Build history of the part. All positions in model axes, mm. Face numbers are marked on the shaded views. Round coordinates to 2 decimals unless told otherwise and drop trailing zeros. Write each loop counter-clockwise with the first axis right and the second up, starting at its lowest first coordinate (ties: lowest second). Pieces come first, ordered by that corner, then holes. Notation, with made-up numbers: (72.25, -7.5) -> (131.25, -7.5) arc R23 cw to (131.25, 1.5) -> close; hole circle Ø9 at (-34.75, 30.25). An arc over 180 degrees is marked (long way). Answer in a Markdown table with one row per item.
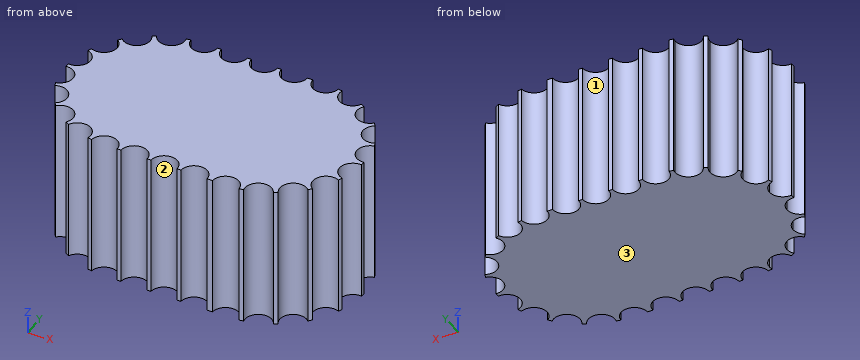
```python
from build123d import *

# Parameters (mm, degrees)
F1_DEPTH = 50.8


with BuildPart() as f1:
    # F0 (on Top) → F1 (new body)
    with BuildSketch(Plane.XY):
        with BuildLine():
            ThreePointArc((-39.4843, 31.75), (-44.0680803662, 26.9908545365), (-48.9958865795, 31.3928125))
            ThreePointArc((-48.9958865795, 31.3928125), (-49.7601296409, 31.2676461581), (-50.5210926164, 31.1238775246))
            ThreePointArc((-50.5210926164, 31.1238775246), (-50.3880618617, 30.485653166), (-50.3434395506, 29.83524071))
            ThreePointArc((-50.3434395506, 29.83524071), (-54.1035181326, 25.1794316985), (-59.4464558449, 27.8753109794))
            ThreePointArc((-59.4464558449, 27.8753109794), (-60.1218, 27.4963065702), (-60.7876995241, 27.1009435801))
            ThreePointArc((-60.7876995241, 27.1009435801), (-60.1220470195, 25.7816931615), (-59.8928066075, 24.321911069))
            ThreePointArc((-59.8928066075, 24.321911069), (-62.859641473, 19.9109029105), (-68.0637222924, 20.9956355589))
            ThreePointArc((-68.0637222924, 20.9956355589), (-68.568711069, 20.4085066075), (-69.0592298315, 19.8092358726))
            ThreePointArc((-69.0592298315, 19.8092358726), (-67.5322058816, 18.0997969887), (-66.9806065702, 15.875))
            ThreePointArc((-66.9806065702, 15.875), (-69.2087580954, 11.8428189452), (-73.808316411, 11.5835766274))
            ThreePointArc((-73.808316411, 11.5835766274), (-74.08204071, 10.8591395506), (-74.3380149087, 10.1282419657))
            ThreePointArc((-74.3380149087, 10.1282419657), (-71.7538504556, 8.4355421952), (-70.7519461581, 5.5133296409))
            ThreePointArc((-70.7519461581, 5.5133296409), (-72.3184192392, 1.9824914708), (-75.987355369, 0.7743673992))
            ThreePointArc((-75.987355369, 0.7743673992), (-75.9968, 0), (-75.987355369, -0.7743673992))
            ThreePointArc((-75.987355369, -0.7743673992), (-72.3184192392, -1.9824914708), (-70.7519461581, -5.5133296409))
            ThreePointArc((-70.7519461581, -5.5133296409), (-71.7538504556, -8.4355421952), (-74.3380149087, -10.1282419657))
            ThreePointArc((-74.3380149087, -10.1282419657), (-74.08204071, -10.8591395506), (-73.808316411, -11.5835766274))
            ThreePointArc((-73.808316411, -11.5835766274), (-69.2087580954, -11.8428189452), (-66.9806065702, -15.875))
            ThreePointArc((-66.9806065702, -15.875), (-67.5322058816, -18.0997969887), (-69.0592298315, -19.8092358726))
            ThreePointArc((-69.0592298315, -19.8092358726), (-68.568711069, -20.4085066075), (-68.0637222924, -20.9956355589))
            ThreePointArc((-68.0637222924, -20.9956355589), (-62.859641473, -19.9109029105), (-59.8928066075, -24.321911069))
            ThreePointArc((-59.8928066075, -24.321911069), (-60.1220470195, -25.7816931615), (-60.7876995241, -27.1009435801))
            ThreePointArc((-60.7876995241, -27.1009435801), (-60.1218, -27.4963065702), (-59.4464558449, -27.8753109794))
            ThreePointArc((-59.4464558449, -27.8753109794), (-54.1035181326, -25.1794316985), (-50.3434395506, -29.83524071))
            ThreePointArc((-50.3434395506, -29.83524071), (-50.3880618617, -30.485653166), (-50.5210926164, -31.1238775246))
            ThreePointArc((-50.5210926164, -31.1238775246), (-49.7601296409, -31.2676461581), (-48.9958865795, -31.3928125))
            ThreePointArc((-48.9958865795, -31.3928125), (-44.0680803662, -26.9908545365), (-39.4843, -31.75))
            Line((-39.4843, -31.75), (-38.0873, -31.75))
            ThreePointArc((-38.0873, -31.75), (-33.3248, -26.9875), (-28.5623, -31.75))
            Line((-28.5623, -31.75), (-27.1653, -31.75))
            ThreePointArc((-27.1653, -31.75), (-22.4028, -26.9875), (-17.6403, -31.75))
            Line((-17.6403, -31.75), (-16.2433, -31.75))
            ThreePointArc((-16.2433, -31.75), (-11.4808, -26.9875), (-6.7183, -31.75))
            Line((-6.7183, -31.75), (-4.7625, -31.75))
            ThreePointArc((-4.7625, -31.75), (-0.1787196338, -26.9908545365), (4.7490865795, -31.3928125))
            ThreePointArc((4.7490865795, -31.3928125), (5.5133296409, -31.2676461581), (6.2742926164, -31.1238775246))
            ThreePointArc((6.2742926164, -31.1238775246), (9.230268618, -25.3599546035), (15.1996558449, -27.8753109794))
            ThreePointArc((15.1996558449, -27.8753109794), (15.875, -27.4963065702), (16.5408995241, -27.1009435801))
            ThreePointArc((16.5408995241, -27.1009435801), (17.3472306164, -20.6736244087), (23.8169222924, -20.9956355589))
            ThreePointArc((23.8169222924, -20.9956355589), (24.321911069, -20.4085066075), (24.8124298315, -19.8092358726))
            ThreePointArc((24.8124298315, -19.8092358726), (23.3718605846, -13.49375), (29.561516411, -11.5835766274))
            ThreePointArc((29.561516411, -11.5835766274), (29.83524071, -10.8591395506), (30.0912149087, -10.1282419657))
            ThreePointArc((30.0912149087, -10.1282419657), (26.5774992344, -4.6863301948), (31.740555369, -0.7743673992))
            ThreePointArc((31.740555369, -0.7743673992), (31.75, 0), (31.740555369, 0.7743673992))
            ThreePointArc((31.740555369, 0.7743673992), (26.5774992344, 4.6863301948), (30.0912149087, 10.1282419657))
            ThreePointArc((30.0912149087, 10.1282419657), (29.83524071, 10.8591395506), (29.561516411, 11.5835766274))
            ThreePointArc((29.561516411, 11.5835766274), (23.3718605846, 13.49375), (24.8124298315, 19.8092358726))
            ThreePointArc((24.8124298315, 19.8092358726), (24.321911069, 20.4085066075), (23.8169222924, 20.9956355589))
            ThreePointArc((23.8169222924, 20.9956355589), (17.3472306164, 20.6736244087), (16.5408995241, 27.1009435801))
            ThreePointArc((16.5408995241, 27.1009435801), (15.875, 27.4963065702), (15.1996558449, 27.8753109794))
            ThreePointArc((15.1996558449, 27.8753109794), (9.230268618, 25.3599546035), (6.2742926164, 31.1238775246))
            ThreePointArc((6.2742926164, 31.1238775246), (5.5133296409, 31.2676461581), (4.7490865795, 31.3928125))
            ThreePointArc((4.7490865795, 31.3928125), (-0.1787196338, 26.9908545365), (-4.7625, 31.75))
            Line((-4.7625, 31.75), (-6.7183, 31.75))
            ThreePointArc((-6.7183, 31.75), (-11.4808, 26.9875), (-16.2433, 31.75))
            Line((-16.2433, 31.75), (-17.6403, 31.75))
            ThreePointArc((-17.6403, 31.75), (-22.4028, 26.9875), (-27.1653, 31.75))
            Line((-27.1653, 31.75), (-28.5623, 31.75))
            ThreePointArc((-28.5623, 31.75), (-33.3248, 26.9875), (-38.0873, 31.75))
            Line((-38.0873, 31.75), (-39.4843, 31.75))
        make_face()
    extrude(amount=F1_DEPTH)


solid = f1.part
```
Q1. Two-plate mould, pull along X, no slides. Class the marked faces 1, 2 and 3: released by +X, released by -X, zero draft, split by the parting line, or undercut.
A:
| item | result |
|---|---|
| face 1 | undercut |
| face 2 | undercut |
| face 3 | zero draft |
Q2. Saw through at B-B on y = 3.5. Write the cut outline in (x, z), plus the area to 3 significant figures.
A:
| item | result |
|---|---|
| outline | (-71.2, 0) -> (26.95, 0) -> (26.95, 50.8) -> (-71.2, 50.8) -> close |
| area | 4,990 mm² |
Q3. Saw through at A-A on x = 0. Write the cut outline in (y, z), plus the area to 3 significant figures.
A:
| item | result |
|---|---|
| outline | (-26.99, 0) -> (26.99, 0) -> (26.99, 50.8) -> (-26.99, 50.8) -> close |
| area | 2,740 mm² |
Q4. Wall check: line 1 (Y direction, x = 24.5, z = 4); line 2 (X direction, y = 28, z = 5.5) (3 decimals); line 3 (X direction, y = 15.5, z = 41). Give the ranges that are in metal, low to high. Write a range as [from, to].
A:
| item | result |
|---|---|
| line 1 | [-20.19, -19.58], [-12.17, 12.17], [19.58, 20.19] |
| line 2 | [-50.711, -47.183], [-41.311, -36.261], [-30.389, -25.339], [-19.467, -14.417], [-8.545, -2.936], [2.936, 6.464] |
| line 3 | [-67, 22.75] |
Q5. Drop a flat-ended pin along its axis: P1, Ø8, axis at y = -20, z = 26.5, coming from the -X side. Give the stop position or say it passes through.
A:
| item | result |
|---|---|
| P1 | x = -69.06 |
